For this review, take the finished solid that the model builds, in its own axes (mm). Coordinates: 2 decimals unless noted, no trailing zeros. One line per question, with ' | ' between items.
from build123d import *

# Parameters (mm, degrees)
F1_W     = 1091
F1_H     = 542
F2_DEPTH = 25


with BuildPart() as f2:
    # F1 (on face) → F2 (new body)
    with BuildSketch(Plane.XY):
        with Locations((545.5, 271)):
            Rectangle(F1_W, F1_H)
        with BuildLine():
            Line((70, 30.25), (50, 30.25))
            ThreePointArc((50, 30.25), (37.5, 42.75), (50, 55.25))
            Line((50, 55.25), (70, 55.25))
            Line((70, 55.25), (70, 50.25))
            Line((70, 50.25), (1021, 50.25))
            Line((1021, 50.25), (1021, 55.25))
            Line((1021, 55.25), (1041, 55.25))
            ThreePointArc((1041, 55.25), (1053.5, 42.75), (1041, 30.25))
            Line((1041, 30.25), (1021, 30.25))
            Line((1021, 30.25), (1021, 35.25))
            Line((1021, 35.25), (70, 35.25))
            Line((70, 35.25), (70, 30.25))
        make_face(mode=Mode.SUBTRACT)
        with BuildLine():
            Line((70, 73), (50, 73))
            ThreePointArc((50, 73), (37.5, 85.5), (50, 98))
            Line((50, 98), (70, 98))
            Line((70, 98), (70, 92))
            Line((70, 92), (1021, 92))
            Line((1021, 92), (1021, 98))
            Line((1021, 98), (1041, 98))
            ThreePointArc((1041, 98), (1053.5, 85.5), (1041, 73))
            Line((1041, 73), (1021, 73))
            Line((1021, 73), (1021, 79))
            Line((1021, 79), (70, 79))
            Line((70, 79), (70, 73))
        make_face(mode=Mode.SUBTRACT)
        with BuildLine():
            Line((70, 115.75), (50, 115.75))
            ThreePointArc((50, 115.75), (37.5, 128.25), (50, 140.75))
            Line((50, 140.75), (70, 140.75))
            Line((70, 140.75), (70, 134.75))
            Line((70, 134.75), (1021, 134.75))
            Line((1021, 134.75), (1021, 140.75))
            Line((1021, 140.75), (1041, 140.75))
            ThreePointArc((1041, 140.75), (1053.5, 128.25), (1041, 115.75))
            Line((1041, 115.75), (1021, 115.75))
            Line((1021, 115.75), (1021, 121.75))
            Line((1021, 121.75), (70, 121.75))
            Line((70, 121.75), (70, 115.75))
        make_face(mode=Mode.SUBTRACT)
        with BuildLine():
            Line((70, 202.061247), (50, 202.061247))
            ThreePointArc((50, 202.061247), (37.5, 214.561247), (50, 227.061247))
            Line((50, 227.061247), (70, 227.061247))
            Line((70, 227.061247), (70, 221.061247))
            Line((70, 221.061247), (1021, 221.061247))
            Line((1021, 221.061247), (1021, 227.061247))
            Line((1021, 227.061247), (1041, 227.061247))
            ThreePointArc((1041, 227.061247), (1053.5, 214.561247), (1041, 202.061247))
            Line((1041, 202.061247), (1021, 202.061247))
            Line((1021, 202.061247), (1021, 208.061247))
            Line((1021, 208.061247), (70, 208.061247))
            Line((70, 208.061247), (70, 202.061247))
        make_face(mode=Mode.SUBTRACT)
        with BuildLine():
            Line((70, 314.938753), (50, 314.938753))
            ThreePointArc((50, 314.938753), (37.5, 327.438753), (50, 339.938753))
            Line((50, 339.938753), (70, 339.938753))
            Line((70, 339.938753), (70, 333.938753))
            Line((70, 333.938753), (1021, 333.938753))
            Line((1021, 333.938753), (1021, 339.938753))
            Line((1021, 339.938753), (1041, 339.938753))
            ThreePointArc((1041, 339.938753), (1053.5, 327.438753), (1041, 314.938753))
            Line((1041, 314.938753), (1021, 314.938753))
            Line((1021, 314.938753), (1021, 320.938753))
            Line((1021, 320.938753), (70, 320.938753))
            Line((70, 320.938753), (70, 314.938753))
        make_face(mode=Mode.SUBTRACT)
        with BuildLine():
            Line((70, 401.25), (50, 401.25))
            ThreePointArc((50, 401.25), (37.5, 413.75), (50, 426.25))
            Line((50, 426.25), (70, 426.25))
            Line((70, 426.25), (70, 420.25))
            Line((70, 420.25), (1021, 420.25))
            Line((1021, 420.25), (1021, 426.25))
            Line((1021, 426.25), (1041, 426.25))
            ThreePointArc((1041, 426.25), (1053.5, 413.75), (1041, 401.25))
            Line((1041, 401.25), (1021, 401.25))
            Line((1021, 401.25), (1021, 407.25))
            Line((1021, 407.25), (70, 407.25))
            Line((70, 407.25), (70, 401.25))
        make_face(mode=Mode.SUBTRACT)
        with BuildLine():
            Line((70, 444), (50, 444))
            ThreePointArc((50, 444), (37.5, 456.5), (50, 469))
            Line((50, 469), (70, 469))
            Line((70, 469), (70, 463))
            Line((70, 463), (1021, 463))
            Line((1021, 463), (1021, 469))
            Line((1021, 469), (1041, 469))
            ThreePointArc((1041, 469), (1053.5, 456.5), (1041, 444))
            Line((1041, 444), (1021, 444))
            Line((1021, 444), (1021, 450))
            Line((1021, 450), (70, 450))
            Line((70, 450), (70, 444))
        make_face(mode=Mode.SUBTRACT)
        with BuildLine():
            Line((70, 486.75), (50, 486.75))
            ThreePointArc((50, 486.75), (37.5, 499.25), (50, 511.75))
            Line((50, 511.75), (70, 511.75))
            Line((70, 511.75), (70, 505.75))
            Line((70, 505.75), (1021, 505.75))
            Line((1021, 505.75), (1021, 511.75))
            Line((1021, 511.75), (1041, 511.75))
            ThreePointArc((1041, 511.75), (1053.5, 499.25), (1041, 486.75))
            Line((1041, 486.75), (1021, 486.75))
            Line((1021, 486.75), (1021, 492.75))
            Line((1021, 492.75), (70, 492.75))
            Line((70, 492.75), (70, 486.75))
        make_face(mode=Mode.SUBTRACT)
    extrude(amount=F2_DEPTH)


solid = f2.part
1) To check wall thickness, follow line 1 along X through (y, z) = (86.5, 18.25); line 2 along X through (y, z) = (412, 2.75). State the ranges of each line that lie inside material, in increasing order. Write a range as [from, to].
Responses:
line 1: [0, 37.54], [1053.46, 1091] | line 2: [0, 37.62], [1053.38, 1091]
2) We need section A-A on x = 338. State how many separate pieces and enclosed holes the cut face has, then the cut area to 3 significant figures.
Responses:
separate pieces: 9 | enclosed holes: 0 | area: 10,900 mm^2
3) Insertion check: pin 1 Ø3 at (y, z) = (95.5, 15) entering from -X. The pin has a flat end and moves straight along its axis. Give the tip position at first contact, or say it passes through.
Responses:
pin 1: x = 0
4) The part is to be moulded in two halves that separate along X. For faces 1 (the flat face through (538, 542, 12)), 2 (the flat face through (552, 320.939, 12)), say which applies: +X half, -X half, draft (parallel to the pull), parting line (faces both ways), or undercut.
Responses:
face 1: draft | face 2: undercut
